from build123d import *

# Parameters (mm, degrees)
SKETCH_1_W                         = 54
SKETCH_1_H                         = 25
SKETCH_1_R                         = 4
SKETCH_1_R_2                       = 1.5
SM_BASE_FLANGE_1_DEPTH             = 2
SM_EDGE_FLANGE_1_STRIP_W           = 10.4732
SM_EDGE_FLANGE_1_STRIP_H           = 2
SM_EDGE_FLANGE_1_STRIP_CUT_DEPTH   = 25
SM_EDGE_FLANGE_1_STRIP_2_W         = 10.4732
SM_EDGE_FLANGE_1_STRIP_2_H         = 2
SM_EDGE_FLANGE_1_STRIP_CUT_2_DEPTH = 25
SM_EDGE_FLANGE_1_DEPTH             = 25
SM_EDGE_FLANGE_1_BEND_DEPTH        = 25
CUT_EXTRUDE_2_DEPTH                = 76.771036683
SKETCH_13_R                        = 4
SKETCH_13_R_2                      = 1.5
CUT_EXTRUDE_3_DEPTH                = 75.619515469


# Sheet-metal steps are written as plain solids
with BuildPart() as part:
    # Sketch 1 → 基体-法兰1 (new body)
    with BuildSketch(Plane.XY):
        with Locations((27, -12.5)):
            Rectangle(SKETCH_1_W, SKETCH_1_H)
        with Locations((27, -12.5)):
            Circle(SKETCH_1_R, mode=Mode.SUBTRACT)
        with Locations((27, -5.5)):
            Circle(SKETCH_1_R_2, mode=Mode.SUBTRACT)
        with Locations((27, -19.5)):
            Circle(SKETCH_1_R_2, mode=Mode.SUBTRACT)
        with Locations((34, -12.5)):
            Circle(SKETCH_1_R_2, mode=Mode.SUBTRACT)
        with Locations((20, -12.5)):
            Circle(SKETCH_1_R_2, mode=Mode.SUBTRACT)
        with Locations((45.5, -12.5)):
            Circle(SKETCH_1_R_2, mode=Mode.SUBTRACT)
        with Locations((8.5, -12.5)):
            Circle(SKETCH_1_R_2, mode=Mode.SUBTRACT)
    extrude(amount=-SM_BASE_FLANGE_1_DEPTH)

    # 边线-法兰1 strip (across the edge) → 边线-法兰1 strip cut (cut)
    with BuildSketch(Plane(origin=(-1, 0, 0), x_dir=(1, 0, 0), z_dir=(0, -1, 0))):
        with Locations((-2.5, -1)):
            Rectangle(SM_EDGE_FLANGE_1_STRIP_W, SM_EDGE_FLANGE_1_STRIP_H)
    extrude(amount=SM_EDGE_FLANGE_1_STRIP_CUT_DEPTH, mode=Mode.SUBTRACT)

    # 边线-法兰1 strip 2 (across the edge) → 边线-法兰1 strip cut 2 (cut)
    with BuildSketch(Plane(origin=(55, -25, 0), x_dir=(-1, 0, 0), z_dir=(0, 1, 0))):
        with Locations((-2.5, -1)):
            Rectangle(SM_EDGE_FLANGE_1_STRIP_2_W, SM_EDGE_FLANGE_1_STRIP_2_H)
    extrude(amount=SM_EDGE_FLANGE_1_STRIP_CUT_2_DEPTH, mode=Mode.SUBTRACT)

    # 边线-法兰1 section (across the edge) → 边线-法兰1 (add)
    with BuildSketch(Plane(origin=(-1, 0, 0), x_dir=(1, 0, 0), z_dir=(0, -1, 0))):
        with BuildLine():
            Line((0, 0.7366), (0, 44.5))
            Line((0, 44.5), (2, 44.5))
            Line((2, 44.5), (2, 0.7366))
            ThreePointArc((2, 0.7366), (2.215745145, 0.215745145), (2.7366, 0))
            Line((2.7366, 0), (2.7366, -2))
            ThreePointArc((2.7366, -2), (0.801531583, -1.198468417), (0, 0.7366))
        make_face()
    extrude(amount=SM_EDGE_FLANGE_1_DEPTH)

    # 边线-法兰1 section 2 (across the edge) → 边线-法兰1 bend (add)
    with BuildSketch(Plane(origin=(55, -25, 0), x_dir=(-1, 0, 0), z_dir=(0, 1, 0))):
        with BuildLine():
            Line((0, 0.7366), (0, 44.5))
            Line((0, 44.5), (2, 44.5))
            Line((2, 44.5), (2, 0.7366))
            ThreePointArc((2, 0.7366), (2.215745145, 0.215745145), (2.7366, 0))
            Line((2.7366, 0), (2.7366, -2))
            ThreePointArc((2.7366, -2), (0.801531583, -1.198468417), (0, 0.7366))
        make_face()
    extrude(amount=SM_EDGE_FLANGE_1_BEND_DEPTH)

    # 草图12 → 切除-拉伸2 (cut, through all)
    with BuildSketch(Plane(origin=(55, 0, 0), x_dir=(0, 0, -1), z_dir=(1, 0, 0))):
        with BuildLine():
            ThreePointArc((-30.009670534, -25), (-42.509670534, -12.5), (-30.009670534, 0))
            Line((-30.009670534, 0), (-44.5, 0))
            Line((-44.5, 0), (-44.5, -25))
            Line((-44.5, -25), (-30.009670534, -25))
        make_face()
    extrude(amount=-CUT_EXTRUDE_2_DEPTH, mode=Mode.SUBTRACT)

    # 草图13 → 切除-拉伸3 (cut, through all)
    with BuildSketch(Plane(origin=(55, 0, 0), x_dir=(0, 0, -1), z_dir=(1, 0, 0))):
        with Locations((-30.009670534, -12.5)):
            Circle(SKETCH_13_R)
        with Locations((-30.009670534, -19.5)):
            Circle(SKETCH_13_R_2)
        with Locations((-37.009670534, -12.5)):
            Circle(SKETCH_13_R_2)
        with Locations((-30.009670534, -5.5)):
            Circle(SKETCH_13_R_2)
        with Locations((-23.009670534, -12.5)):
            Circle(SKETCH_13_R_2)
        with Locations((-11.409670534, -12.5)):
            Circle(SKETCH_13_R_2)
    extrude(amount=-CUT_EXTRUDE_3_DEPTH, mode=Mode.SUBTRACT)


solid = part.part
Input: part model. Units: mm. Frame: model coordinates. Give positions to 0.01 mm unless a question says otherwise; leave off trailing zeros. Order: outer loops, then holes, each group sorted by start corner. A loop starts at its lowest first (then second) coordinate and runs counter-clockwise, first axis right, second up.
Q1. Section A-A on x = 27. Output: boundary loops of the cut face in (y, z).
Checked values:
outline: (-25, -2) - (-21, -2) - (-21, 0) - (-25, 0) - close; (-18, -2) - (-16.5, -2) - (-16.5, 0) - (-18, 0) - close; (-8.5, -2) - (-7, -2) - (-7, 0) - (-8.5, 0) - close; (-4, -2) - (0, -2) - (0, 0) - (-4, 0) - close
Q2. Contact query for flat-ended pins moving along their axis: pin 1 Ø1.8 at (x, y) = (45.5, -12.5) entering from +Z; pin 2 Ø4 at (x, y) = (22.5, -15) entering from +Z. Output: stop coordinate, or through.
Checked values:
pin 1: passes through
pin 2: stops at z = 0
Q3. Section B-B on z = 7. Output: boundary loops of the cut face in (x, y), and give its area (3 significant figures).
Checked values:
outline: (-1, -25) - (1, -25) - (1, 0) - (-1, 0) - close; (53, -25) - (55, -25) - (55, 0) - (53, 0) - close
area: 100 mm2
Q4. Section D-D on y = -12.5. State how many separate pieces and enclosed holes the cut face has, and give its area (3 significant figures).
Checked values:
separate pieces: 14
enclosed holes: 0
area: 171 mm2
Q5. Section C-C on x = 20. Output: boundary loops of the cut face in (y, z), and give its area (3 significant figures).
Checked values:
outline: (-25, -2) - (-14, -2) - (-14, 0) - (-25, 0) - close; (-11, -2) - (0, -2) - (0, 0) - (-11, 0) - close
area: 44.0 mm2
Q6. Draft query along Z for faces 1 (the cylindrical face through (54.014, -11.299, 26.194)), 2 (the cylindrical face through (0.01, -5.43, 31.51)), 3 (the flat face through (53, -13, 17)), 4 (the flat face through (32, -12, 0)). Return one class per face: +Z half, -Z half, draft (parallel to the pull), parting line (faces both ways), or undercut.
Checked values:
face 1: undercut
face 2: undercut
face 3: draft
face 4: +Z half
Q7. Ray query, probe 1 along Y at (x, z) = (27, -0.5); probe 2 along X at (y, z) = (-2.25, 23.5); probe 3 along Z at (x, y) = (50.5, -9.5). Return the intervals inside material, ascending.
Checked values:
probe 1: y = -25 to -21, -18 to -16.5, -8.5 to -7, -4 to 0
probe 2: x = -1 to 1, 53 to 55
probe 3: z = -2 to 0
